Answer from the drawing. Dimensions are ordinates in mm from the lowest x, y and z of the part. A direction names the side the tool comes from. Coordinates: 2 decimals unless noted, no trailing zeros. Write each loop counter-clockwise with the first axis right and the second up, starting at its lowest first coordinate (ties: lowest second). Pieces come first, ordered by that corner, then holes.
(1) Which of the six approach directions +Z, -Z, +X, -X, +Y, -Y give full straight-line access (tool end or side, diameter ignored) to the marked faces 1, 2 and 3?
(2) Straight lines are drawn through the part: line 1 (X direction, y = 23.5, z = 18.5); line 2 (Z direction, x = 13, y = 2.75); line 3 (Y direction, x = 20.25, z = 67). For each, find the intervals that lie inside material, in ascending order.
(3) Given P1, Ø5, axis at x = 3.5, y = 11.5, coming from the +Z side; P2, Ø2.5, axis at y = 23.5, z = 45, coming from the -X side; P3, Ø4, axis at x = 18, z = 43, coming from the +Y side, each flat-ended and moving along its own axis, determine where each tip first touches the part or whether it passes through.
(4) The part is cut by section D-D on z = 96.2. Determine the outline of the cut face in (x, y).
(5) The part is cut by section C-C on y = 8. Determine the outline of the cut face in (x, z).
(6) The part is cut by section A-A on z = 49.5. Determine the outline of the cut face in (x, y), plus the area to 4 significant figures.
(7) The part is cut by section B-B on x = 11.5. Determine the outline of the cut face in (y, z), plus the area to 3 significant figures.
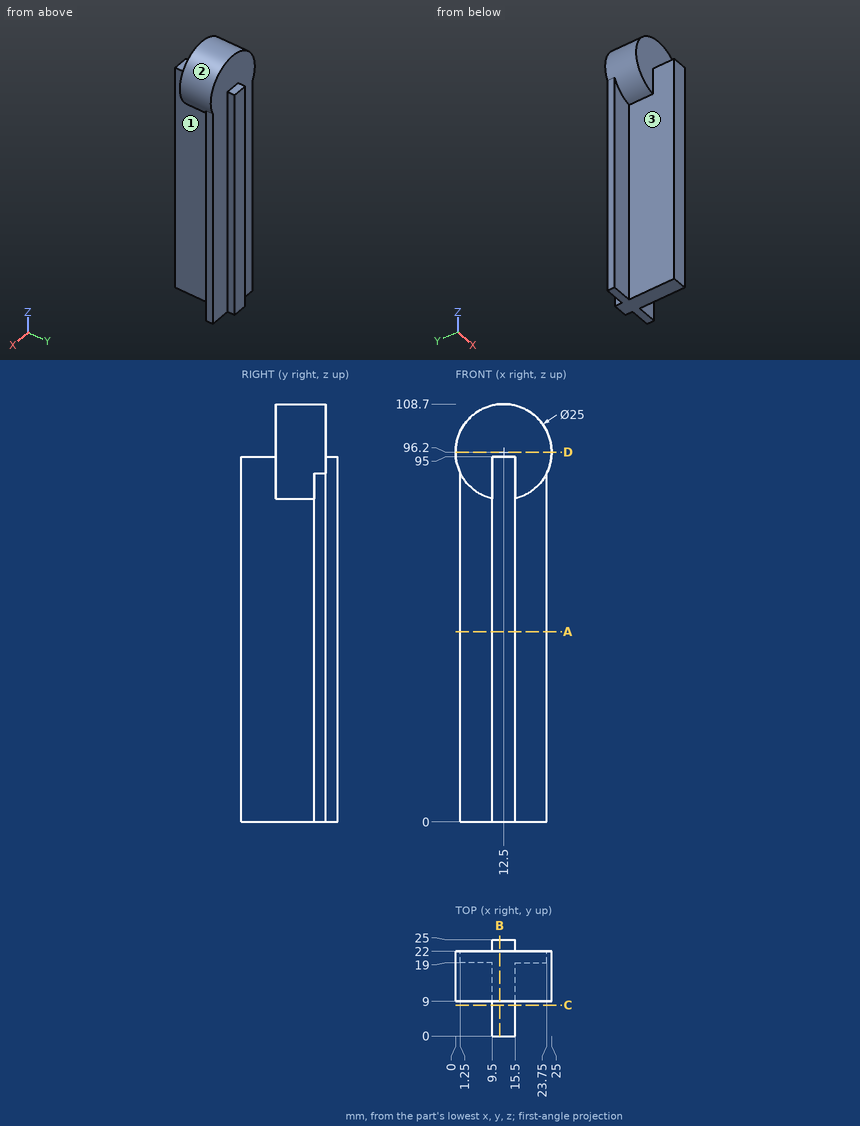
Model answer:
1. face 1: -Z, +X, -Y
1. face 2: -Y
1. face 3: -Z, -X, -Y
2. line 1: x = 9.5 to 15.5
2. line 2: z = 0 to 95
2. line 3: y = 19 to 22
3. P1: stops at z = 106.88
3. P2: stops at x = 9.5
3. P3: stops at y = 22
4. outline: (0, 9) - (25, 9) - (25, 22) - (0, 22) - close
5. outline: (9.5, 0) - (15.5, 0) - (15.5, 95) - (9.5, 95) - close
6. outline: (1.25, 19) - (9.5, 19) - (9.5, 0) - (15.5, 0) - (15.5, 19) - (23.75, 19) - (23.75, 22) - (15.5, 22) - (15.5, 25) - (9.5, 25) - (9.5, 22) - (1.25, 22) - close
6. area: 199.5 mm2
7. outline: (0, 0) - (25, 0) - (25, 95) - (22, 95) - (22, 108.66) - (9, 108.66) - (9, 95) - (0, 95) - close
7. area: 2,550 mm2
